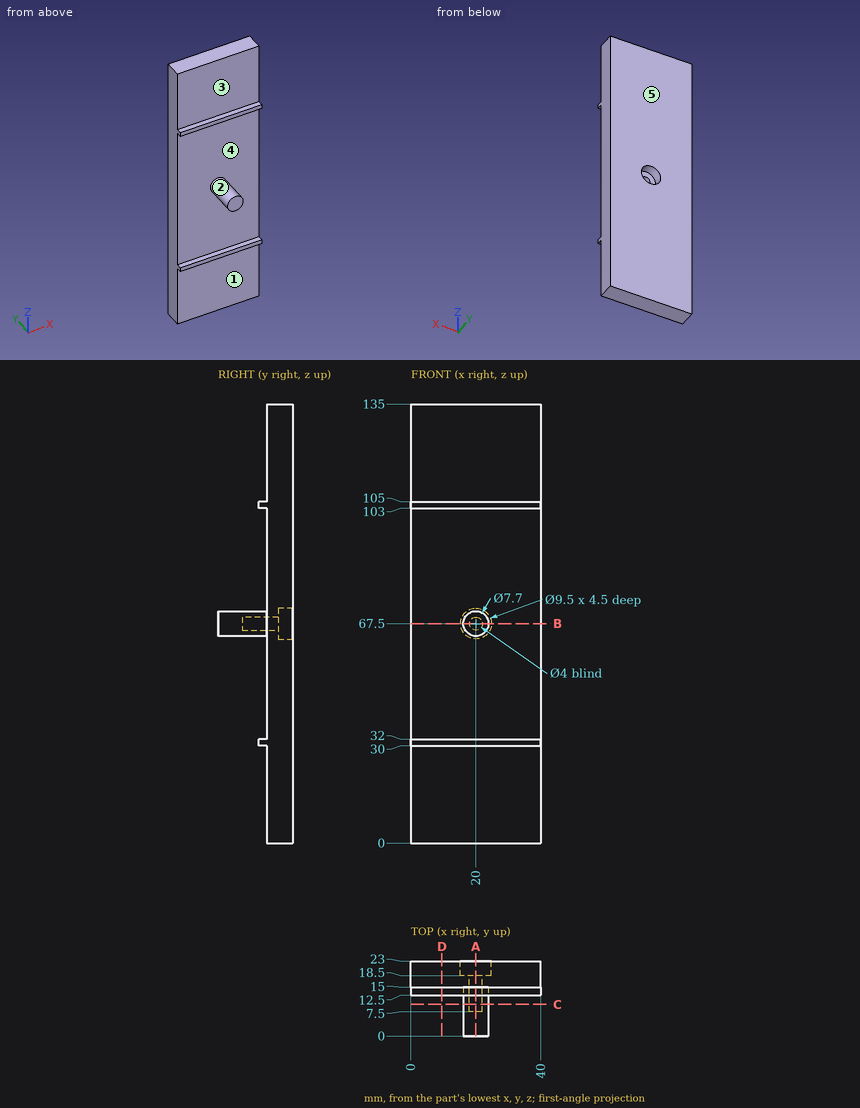
Answer from the drawing. Dimensions are ordinates in mm from the lowest x, y and z of the part. A direction names the side the tool comes from. Give positions to 0.01 mm unless a question says otherwise; leave off trailing zeros. Order: outer loops, then holes, each group sorted by start corner. A loop starts at its lowest first (then second) coordinate and runs counter-clockwise, first axis right, second up.
Item 1: For a pull along Z with two mould halves and no side action, classify the marked faces 4 and 5 as pulls with the +Z half, pulls with the -Z half, needs draft (parallel to the pull), parting line crosses it, or undercut.
From the geometry:
face 4: undercut
face 5: needs draft
Item 2: Find the intervals of material crossed by probe 1 along X at (y, z) = (14.25, 67.5); probe 2 along X at (y, z) = (21.65, 67.5); probe 3 along Y at (x, z) = (26, 70), in increasing order.
From the geometry:
probe 1: x = 16.15 to 18, 22 to 23.85
probe 2: x = 0 to 15.25, 24.75 to 40
probe 3: y = 15 to 23
Item 3: The part is cut by section C-C, the plane y = 9.75. Give the vertices of the cut face in (x, z), and give its area (3 significant figures).
From the geometry:
outline: circle Ø7.7 at (20, 67.5); hole circle Ø4 at (20, 67.5)
area: 34.0 mm2
Item 4: The part is cut by section B-B, the plane z = 67.5. Give the vertices of the cut face in (x, y).
From the geometry:
outline: (0, 15) - (16.15, 15) - (16.15, 0) - (23.85, 0) - (23.85, 15) - (40, 15) - (40, 23) - (24.75, 23) - (24.75, 18.5) - (22, 18.5) - (22, 7.5) - (18, 7.5) - (18, 18.5) - (15.25, 18.5) - (15.25, 23) - (0, 23) - close
Item 5: The part is cut by section A-A, the plane x = 20. Give the vertices of the cut face in (y, z), and give its area (3 significant figures).
From the geometry:
outline: (0, 63.65) - (15, 63.65) - (15, 32) - (12.5, 32) - (12.5, 30) - (15, 30) - (15, 0) - (23, 0) - (23, 62.75) - (18.5, 62.75) - (18.5, 65.5) - (7.5, 65.5) - (7.5, 69.5) - (18.5, 69.5) - (18.5, 72.25) - (23, 72.25) - (23, 135) - (15, 135) - (15, 105) - (12.5, 105) - (12.5, 103) - (15, 103) - (15, 71.35) - (0, 71.35) - close
area: 1,120 mm2
Item 6: The part is cut by section D-D, the plane x = 9.5. Give the vertices of the cut face in (y, z).
From the geometry:
outline: (12.5, 30) - (15, 30) - (15, 0) - (23, 0) - (23, 135) - (15, 135) - (15, 105) - (12.5, 105) - (12.5, 103) - (15, 103) - (15, 32) - (12.5, 32) - close
Item 7: Which of the six approach directions +Z, -Z, +X, -X, +Y, -Y give full straight-line access (tool end or side, diameter ignored) to the marked faces 1, 2 and 3?
From the geometry:
face 1: -Z, +X, -X, -Y
face 2: -Y
face 3: +Z, +X, -X, -Y
Item 8: Given pin 1 Ø4.5 at (x, z) = (20.5, 67) entering from +Y; pin 2 Ø2 at (x, z) = (26.5, 104) entering from -Y; pin 3 Ø1.5 at (x, z) = (21, 95.5) entering from -Y; pin 4 Ø1 at (x, y) = (15.5, 11) entering from -Z, each flat-ended and moving along its own axis, determine where each tip first touches the part or whether it passes through.
From the geometry:
pin 1: stops at y = 18.5
pin 2: stops at y = 12.5
pin 3: stops at y = 15
pin 4: passes through
